from build123d import *

# Parameters (mm, degrees)
SKETCH1_R           = 1.6
BOSS_EXTRUDE1_DEPTH = 4.5
FILLET1_R           = 4
FILLET2_R           = 6
FILLET3_R           = 3
CHAMFER1_SIZE       = 2
CHAMFER1_SIZE2      = 1.419615628


with BuildPart() as part:
    # Sketch1 → Boss-Extrude1 (new body)
    # profile 1 of 2: a face of its own
    with BuildSketch(Plane(origin=(0, 0, 0), x_dir=(1, 0, 0), z_dir=(0, 1, 0))):
        with BuildLine():
            Line((3.5, 0), (3.5, 18))
            ThreePointArc((3.5, 18), (0, 21.5), (-3.5, 18))
            Line((-3.5, 18), (-3.5, 0))
            ThreePointArc((-3.5, 0), (0, -3.5), (3.5, 0))
        make_face()
        with Locations(Location((0, 0, 0), (0, 0, 270))):
            Circle(SKETCH1_R, mode=Mode.SUBTRACT)
    # profile 2 of 2: a face of its own
    with BuildSketch(Plane(origin=(0, 0, 0), x_dir=(1, 0, 0), z_dir=(0, 1, 0))):
        with BuildLine():
            Line((24.303924048, 30.570527133), (-1.197070502, 21.288924173))
            ThreePointArc((-1.197070502, 21.288924173), (2.007517527, 20.867032155), (3.5, 18))
            Line((3.5, 18), (3.5, 16.613451389))
            Line((3.5, 16.613451389), (22.597274425, 23.564290835))
            Line((22.597274425, 23.564290835), (25.675455715, 15.107057248))
            Line((25.675455715, 15.107057248), (22.721032456, 14.586112715))
            Line((22.721032456, 14.586112715), (25.221032456, 12.488363637))
            Line((25.221032456, 12.488363637), (30.543696603, 13.426892935))
            Line((30.543696603, 13.426892935), (24.303924048, 30.570527133))
        make_face()
    extrude(amount=BOSS_EXTRUDE1_DEPTH)

    # Fillet1
    fillet1_edges = [part.edges().sort_by_distance(p)[0] for p in [
        (3.5, 2.25, -16.613451389),
    ]]
    fillet(fillet1_edges, radius=FILLET1_R)

    # Fillet2
    fillet2_edges = [part.edges().sort_by_distance(p)[0] for p in [
        (24.303924048, 2.25, -30.570527133),
        (22.597274425, 2.25, -23.564290835),
    ]]
    fillet(fillet2_edges, radius=FILLET2_R)

    # Fillet3
    fillet3_edges = [part.edges().sort_by_distance(p)[0] for p in [
        (30.543696603, 2.25, -13.426892935),
    ]]
    fillet(fillet3_edges, radius=FILLET3_R)

    # Chamfer1
    chamfer1_edges = [part.edges().sort_by_distance(p)[0] for p in [
        (22.721032456, 2.25, -14.586112715),
    ]]
    chamfer1_side = [part.faces().sort_by_distance(p)[0] for p in [
        (24.198244085, 2.25, -14.846584982),
    ]]
    chamfer(chamfer1_edges, length=CHAMFER1_SIZE, length2=CHAMFER1_SIZE2, reference=chamfer1_side[0])


solid = part.part
Could you check a few things on this model? Use its own coordinates, in mm. A direction names the side the tool comes from. Round coordinates to 2 decimals unless told otherwise and drop trailing zeros. Order: outer loops, then holes, each group sorted by start corner. A loop starts at its lowest first (then second) coordinate and runs counter-clockwise, first axis right, second up.
Q1. Imagine slicing it at B-B, the plane x = 1. List the corners of the cut face in (y, z) for me, then the cut area to 3 significant figures.
Geometry says:
outline: (0, -22.09) - (4.5, -22.09) - (4.5, -1.25) - (0, -1.25) - close; (0, 1.25) - (4.5, 1.25) - (4.5, 3.35) - (0, 3.35) - close
area: 103 mm2
Q2. Thinking about a two-plate mould opening in X: for faces 1 (the face through (-2.85, 2.22, -20.03)), 2 (the face through (-0.1, 2.2, 3.5)), 3 (the face through (25.155, 2.218, -16.536)), 4 (the face through (29.08, 2.28, -14.23)), which applies, released by +X, released by -X, zero draft, split by the parting line, or undercut?
Geometry says:
face 1: released by -X
face 2: split by the parting line
face 3: undercut
face 4: released by +X
Q3. I'm going to push flat-ended pins straight in: P1, Ø2, axis at y = 2.5, z = 0, coming from the +X side; P2, Ø1.5, axis at y = 1, z = -19.5, coming from the -X side. Where does each tip first touch, or does it pass through?
Geometry says:
P1: stops at x = 3.5
P2: stops at x = -3.42
Q4. Please list where these lines run through material, in increasing order: probe 1 along X at (y, z) = (1.8, 0); probe 2 along X at (y, z) = (3.55, -9.5); probe 3 along Z at (x, y) = (15.5, 2.3).
Geometry says:
probe 1: x = -3.5 to -1.6, 1.6 to 3.5
probe 2: x = -3.5 to 3.5
probe 3: z = -27.37 to -20.98
Q5. Imagine slicing it at A-A, the plane y = 4.05. List the corners of the cut face in (x, z) for me.
Geometry says:
outline: (-3.5, -18) arc R3.5 ccw to (-1.2, -21.29) - (18.67, -28.52) arc R6 ccw to (26.36, -24.93) - (29.32, -16.79) arc R3 ccw to (27.02, -12.81) - (25.22, -12.49) - (23.81, -13.67) - (24.69, -14.93) - (25.68, -15.11) - (24.65, -17.93) arc R6 cw to (16.96, -21.51) - (6.13, -17.57) arc R4 cw to (3.5, -13.81) - (3.5, 0) arc R3.5 ccw to (-3.5, 0) - close; hole circle Ø3.2 at (0, 0)
Q6. Imagine slicing it at C-C, the plane z = -7.5. List the corners of the cut face in (x, y) for me.
Geometry says:
outline: (-3.5, 0) - (3.5, 0) - (3.5, 4.5) - (-3.5, 4.5) - close
Q7. Imagine slicing it at D-D, the plane x = 10. List the corners of the cut face in (y, z) for me, then the cut area to 3 significant figures.
Geometry says:
outline: (0, -25.36) - (4.5, -25.36) - (4.5, -18.98) - (0, -18.98) - close
area: 28.7 mm2
Q8. Which directions (+Z, -Z, +X, -X, +Y, -Y) give clear straight access to the entire face, cutting with the end or side of a thin tool? Please do faces 5 (the face through (9, 4.5, -19)), 6 (the face through (24.24, 2.22, -14.29)), 7 (the face through (24.505, 2.218, -13.089)).
Geometry says:
face 5: +Z, -Z, +X, -X, +Y
face 6: +Y, -Y
face 7: +Z, +Y, -Y
